```python
from build123d import *

# Parameters (mm, degrees)
EXTRUDE1_DEPTH      = 12.7
SKETCH27_R          = 33.3375
EXTRUDE3_DEPTH      = 38.1
SKETCH29_R          = 4.7879
SKETCH29_R_2        = 25.2349
CUT_EXTRUDE5_DEPTH  = 50.8
SKETCH41_R          = 25.2349
SKETCH41_R_2        = 22.0599
BOSS_EXTRUDE1_DEPTH = 596.9
SKETCH42_R          = 22.5679
BOSS_EXTRUDE2_DEPTH = 12.7


with BuildPart() as part:
    # Sketch1 → Extrude1 (new body)
    with BuildSketch(Plane.XY):
        with BuildLine():
            Line((-98.171, 30.1625), (-98.171, -30.1625))
            ThreePointArc((-98.171, -30.1625), (-94.990618984, -37.840618984), (-87.3125, -41.021))
            Line((-87.3125, -41.021), (-42.161003408, -41.021))
            ThreePointArc((-42.161003408, -41.021), (-35.938003408, -39.353552176), (-31.382451232, -34.798))
            Line((-31.382451232, -34.798), (-15.342939066, -7.01675))
            ThreePointArc((-15.342939066, -7.01675), (0, 1.8415), (15.342939066, -7.01675))
            Line((15.342939066, -7.01675), (31.382451232, -34.798))
            ThreePointArc((31.382451232, -34.798), (35.938003408, -39.353552176), (42.161003408, -41.021))
            Line((42.161003408, -41.021), (87.3125, -41.021))
            ThreePointArc((87.3125, -41.021), (94.990618984, -37.840618984), (98.171, -30.1625))
            Line((98.171, -30.1625), (98.171, 30.1625))
            ThreePointArc((98.171, 30.1625), (94.990618984, 37.840618984), (87.3125, 41.021))
            Line((87.3125, 41.021), (-87.3125, 41.021))
            ThreePointArc((-87.3125, 41.021), (-94.990618984, 37.840618984), (-98.171, 30.1625))
        make_face()
    extrude(amount=-EXTRUDE1_DEPTH)

    # Sketch27 → Extrude3 (add)
    with BuildSketch(Plane.XY):
        with Locations(Location((-57.15, 0, 0), (0, 0, 180))):
            Circle(SKETCH27_R)
        with Locations(Location((57.15, 0, 0), (0, 0, 180))):
            Circle(SKETCH27_R)
    extrude(amount=EXTRUDE3_DEPTH)

    # Sketch29 → Cut-Extrude5 (cut, symmetric)
    with BuildSketch(Plane.XY):
        with Locations((-87.3125, -30.1625)):
            Circle(SKETCH29_R)
        with Locations((87.3125, -30.1625)):
            Circle(SKETCH29_R)
        with Locations((87.3125, 30.1625)):
            Circle(SKETCH29_R)
        with Locations((-87.3125, 30.1625)):
            Circle(SKETCH29_R)
        with Locations((57.15, 0)):
            Circle(SKETCH29_R_2)
        with Locations((-57.15, 0)):
            Circle(SKETCH29_R_2)
    extrude(amount=CUT_EXTRUDE5_DEPTH, both=True, mode=Mode.SUBTRACT)

    # Sketch41 → Boss-Extrude1 (add)
    # profile 1 of 2: a face of its own
    with BuildSketch(Plane(origin=(0, 0, 38.1), x_dir=(-1, 0, 0), z_dir=(0, 0, -1))):
        with Locations(Location((-57.15, 0, 0), (0, 0, 180))):
            Circle(SKETCH41_R)
        with Locations((-57.15, 0)):
            Circle(SKETCH41_R_2, mode=Mode.SUBTRACT)
    # profile 2 of 2: a face of its own
    with BuildSketch(Plane(origin=(0, 0, 38.1), x_dir=(-1, 0, 0), z_dir=(0, 0, -1))):
        with Locations(Location((57.15, 0, 0), (0, 0, 180))):
            Circle(SKETCH41_R)
        with Locations((57.15, 0)):
            Circle(SKETCH41_R_2, mode=Mode.SUBTRACT)
    extrude(amount=BOSS_EXTRUDE1_DEPTH)

    # Sketch42 → Boss-Extrude2 (add)
    with BuildSketch(Plane(origin=(0, 0, -558.8), x_dir=(-1, 0, 0), z_dir=(0, 0, -1))):
        with BuildLine():
            Line((57.15, 31.75), (-57.15, 31.75))
            ThreePointArc((-57.15, 31.75), (-69.446722124, 29.272053652), (-79.824035261, 22.225))
            Line((-79.824035261, 22.225), (-95.25, 22.225))
            Line((-95.25, 22.225), (-95.25, -22.225))
            Line((-95.25, -22.225), (-79.824035261, -22.225))
            ThreePointArc((-79.824035261, -22.225), (-69.446722124, -29.272053652), (-57.15, -31.75))
            Line((-57.15, -31.75), (57.15, -31.75))
            ThreePointArc((57.15, -31.75), (69.446722124, -29.272053652), (79.824035261, -22.225))
            Line((79.824035261, -22.225), (95.25, -22.225))
            Line((95.25, -22.225), (95.25, 22.225))
            Line((95.25, 22.225), (79.824035261, 22.225))
            ThreePointArc((79.824035261, 22.225), (69.446722124, 29.272053652), (57.15, 31.75))
        make_face()
        with Locations((-57.15, 0)):
            Circle(SKETCH42_R, mode=Mode.SUBTRACT)
        with Locations((57.15, 0)):
            Circle(SKETCH42_R, mode=Mode.SUBTRACT)
    extrude(amount=-BOSS_EXTRUDE2_DEPTH)


solid = part.part
```
The listing builds one solid part. Answer for the finished solid, in the listing's coordinates (mm). A direction names the side the tool comes from. Round coordinates to 2 decimals unless told otherwise and drop trailing zeros. Order: outer loops, then holes, each group sorted by start corner. A loop starts at its lowest first (then second) coordinate and runs counter-clockwise, first axis right, second up. Notation, with made-up numbers: (2, 87.5) -> (42, 87.5) arc R4 cw to (42, 92.5) -> close; hole circle Ø4 at (-20, 23.25). An arc over 180 degrees is marked (long way). Answer as CSV lines item,"result". Start each with the question number.
(1) A tool of negligible diameter and unlimited length cuts with its end or side. For faces 1 (the face through (35.86, -39.31, -6.26)), 2 (the face through (87, 22.225, -553)), 3 (the face through (-75.07, -28.11, 18.78)), from which of +Z, -Z, +X, -X, +Y, -Y can it reach the whole face along a straight path? Write none if from no direction.
(2) The part is cut by section C-C (x = -68). Determine the outline of the cut face in (y, z), then the cut area to 3 significant figures.
(3) Find the intervals of material crossed by probe 1 along Z at (x, y) = (27.5, 13); probe 2 along Z at (x, y) = (0, 6.5); probe 3 along X at (y, z) = (-10, -348), in increasing order. Write a range as from..to.
(4) For a pull along Z with two mould halves and no side action, classify faces 4 (the face through (69.61, -29.203, -552.539)), 5 (the face through (81.22, -7.58, -275.67)) as +Z half, -Z half, draft (parallel to the pull), parting line (faces both ways), or undercut.
(5) The part is cut by section A-A (z = -295.5). Determine the outline of the cut face in (x, y), then the cut area to 3 significant figures.
(6) The part is cut by section B-B (x = -1.5). Determine the outline of the cut face in (y, z), then the cut area to 3 significant figures.
(7) Flat-ended cylindrical pins translate along their axes: pin 1 Ø4 at (x, z) = (-91, -550.5) entering from +Y (3 decimals); pin 2 Ø4 at (x, z) = (88, -551.5) entering from -Y (3 decimals); pin 3 Ø6 at (x, z) = (36, -461.5) entering from -Y; pin 4 Ø7.5 at (x, y) = (87.31, -30.16) entering from +Z. Find the tip coordinate at first contact, or state that the pin passes through.
Evaluation:
1,face 1,"+Z, -Z, -Y"
1,face 2,"-Z, +X, +Y"
1,face 3,"+Z"
2,outline,"(-41.02, -12.7) -> (-22.78, -12.7) -> (-22.78, -546.1) -> (-29.84, -546.1) -> (-29.84, -558.8) -> (-19.21, -558.8) -> (-19.21, 38.1) -> (-31.52, 38.1) -> (-31.52, 0) -> (-41.02, 0) -> close; (19.21, -558.8) -> (29.84, -558.8) -> (29.84, -546.1) -> (22.78, -546.1) -> (22.78, -12.7) -> (41.02, -12.7) -> (41.02, 0) -> (31.52, 0) -> (31.52, 38.1) -> (19.21, 38.1) -> close"
2,area,"5,580 mm²"
3,probe 1,"-558.8..-546.1, -12.7..38.1"
3,probe 2,"-558.8..-546.1, -12.7..0"
3,probe 3,"-80.32..-76.81, -37.49..-33.98, 33.98..37.49, 76.81..80.32"
4,face 4,"draft"
4,face 5,"undercut"
5,outline,"circle Ø50.47 at (-57.15, 0); circle Ø50.47 at (57.15, 0); hole circle Ø44.12 at (-57.15, 0); hole circle Ø44.12 at (57.15, 0)"
5,area,"943 mm²"
6,outline,"(-31.75, -558.8) -> (31.75, -558.8) -> (31.75, -546.1) -> (-31.75, -546.1) -> close; (1.78, -12.7) -> (41.02, -12.7) -> (41.02, 0) -> (1.78, 0) -> close"
6,area,"1,300 mm²"
7,pin 1,"y = 22.225"
7,pin 2,"y = -22.225"
7,pin 3,"y = -17.53"
7,pin 4,"through"
